```python
from build123d import *

# Parameters (mm, degrees)
PAD003_DEPTH = 2
SKETCH014_R  = 1.5
PAD005_DEPTH = 8
SKETCH015_R  = 2.45
PAD006_DEPTH = 4


with BuildPart() as part:
    # Sketch012 → Pad003 (new body)
    with BuildSketch(Plane.XY):
        Polygon((-15, 75.3), (53.6, 75.3), (53.6, 24.12132), (53.6, 18), (43.6, 18), (43.6, 22), (-5, 22), (-5, 18), (-15, 18), (-15, 22), align=None)
        with BuildLine():
            Line((-13, 73.3), (-3.668627, 73.3))
            ThreePointArc((-3.668627, 73.3), (0.3, 68.8), (4.268627, 73.3))
            Line((4.268627, 73.3), (51.6, 73.3))
            Line((51.6, 73.3), (51.6, 61.568627))
            ThreePointArc((51.6, 61.568627), (47.1, 57.6), (51.6, 53.631373))
            Line((51.6, 53.631373), (51.6, 33.568627))
            ThreePointArc((51.6, 33.568627), (47.1, 29.6), (51.6, 25.631373))
            Line((51.6, 25.631373), (51.6, 24))
            Line((51.6, 24), (2.968627, 24))
            ThreePointArc((2.968627, 24), (-1, 28.5), (-4.968627, 24))
            Line((-4.968627, 24), (-13, 24))
            Line((-13, 24), (-13, 73.3))
        make_face(mode=Mode.SUBTRACT)
    extrude(amount=PAD003_DEPTH)

    # Sketch014 → Pad005 (join)
    with BuildSketch(Plane.XY):
        with Locations((0.3, 72.8)):
            Circle(SKETCH014_R)
        with Locations((51.1, 57.6)):
            Circle(SKETCH014_R)
        with Locations((51.1, 29.6)):
            Circle(SKETCH014_R)
        with Locations((-1, 24.5)):
            Circle(SKETCH014_R)
    extrude(amount=-PAD005_DEPTH)

    # Sketch015 → Pad006 (join)
    with BuildSketch(Plane.XY):
        with Locations((0.3, 72.8)):
            Circle(SKETCH015_R)
        with Locations((51.1, 57.6)):
            Circle(SKETCH015_R)
        with Locations((51.1, 29.6)):
            Circle(SKETCH015_R)
        with Locations((-1, 24.5)):
            Circle(SKETCH015_R)
    extrude(amount=-PAD006_DEPTH)


solid = part.part
```
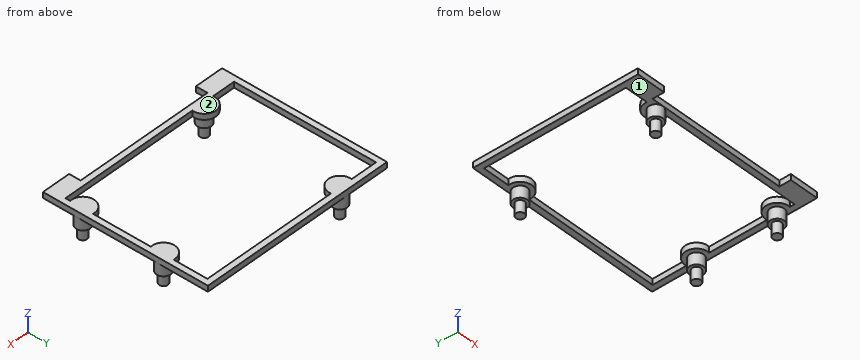
CAD build for the part. Positions are in the model's coordinates, mm. Face numbers are marked on the shaded views. A direction names the side the tool comes from. Coordinates: 2 decimals unless noted, no trailing zeros. Write each loop counter-clockwise with the first axis right and the second up, starting at its lowest first coordinate (ties: lowest second). Pieces come first, ordered by that corner, then holes.
(1) 3-axis set-ups, long thin cutter, end or side, ignore diameter. For the marked faces 1 and 2: which of +Z, -Z, +X, -X, +Y, -Y reach the whole face in a straight line?
(2) Cut at A-A, the plane x = 22.5. List the corners of the cut face in (y, z).
(3) Drill centre lines: probe 1 along Y at (x, z) = (16.5, 0.75); probe 2 along Y at (x, z) = (-10, 0.5); probe 3 along X at (y, z) = (42, 1.25). Where is each one in solid material? Low to high.
(4) Cut at C-C, the plane z = -7. List the corners of the cut face in (x, y), and give its area (3 significant figures).
(5) Cut at D-D, the plane y = 57.6. List the corners of the cut face in (x, z).
(6) Flat gauge pins, fed straight in: pin 1 (4 mm diameter, centred on x = 39, z = -3, fed in from +Y); pin 2 (8 mm diameter, centred on x = 5, y = 29, fed in from -Z); pin 3 (1.6 mm diameter, centred on x = 25, z = 0.5, fed in from -Y). Where does each tip first touch, or does it go through?
(7) Cut at B-B, the plane y = 37. List the corners of the cut face in (x, z).
Geometry says:
1. face 1: -Z
1. face 2: +Z, +X, -X, +Y, -Y
2. outline: (22, 0) - (24, 0) - (24, 2) - (22, 2) - close; (73.3, 0) - (75.3, 0) - (75.3, 2) - (73.3, 2) - close
3. probe 1: y = 22 to 24, 73.3 to 75.3
3. probe 2: y = 18 to 24, 73.3 to 75.3
3. probe 3: x = -15 to -13, 51.6 to 53.6
4. outline: circle Ø3 at (-1, 24.5); circle Ø3 at (0.3, 72.8); circle Ø3 at (51.1, 29.6); circle Ø3 at (51.1, 57.6)
4. area: 28.3 mm2
5. outline: (-15, 0) - (-13, 0) - (-13, 2) - (-15, 2) - close; (47.1, 0) - (48.65, 0) - (48.65, -4) - (49.6, -4) - (49.6, -8) - (52.6, -8) - (52.6, -4) - (53.55, -4) - (53.55, 0) - (53.6, 0) - (53.6, 2) - (47.1, 2) - close
6. pin 1: passes through
6. pin 2: stops at z = 0
6. pin 3: stops at y = 22
7. outline: (-15, 0) - (-13, 0) - (-13, 2) - (-15, 2) - close; (51.6, 0) - (53.6, 0) - (53.6, 2) - (51.6, 2) - close
